Can you work these out from the model? Positions are in its coordinate system, mm. A direction names the side the tool comes from. Give positions to 0.01 mm unless a question says otherwise; leave off trailing zeros. Answer as a JSON object with one key per item and string values.
```python
from build123d import *

# Parameters (mm, degrees)
SKETCH1_W                = 127
SKETCH1_H                = 57.15
BOSS_EXTRUDE1_DEPTH      = 6.35
BOSS_EXTRUDE2_DEPTH      = 22.225
BOSS_EXTRUDE2_DEPTH_BACK = 22.225
SKETCH3_R                = 22.225
SKETCH4_R                = 12.7
CUT_EXTRUDE2_DEPTH       = 83.611035128
CUT_EXTRUDE2_DRAFT       = -7.5
BOSS_EXTRUDE3_DEPTH      = 6.35
CHAMFER1_SIZE            = 3.175
CHAMFER1_SIZE2           = 3.687920954
FILLET1_R                = 2.0955


with BuildPart() as part:
    # Sketch1 → Boss-Extrude1 (new body)
    with BuildSketch(Plane(origin=(0, 0, 0), x_dir=(1, 0, 0), z_dir=(0, 1, 0))):
        Rectangle(SKETCH1_W, SKETCH1_H)
    extrude(amount=BOSS_EXTRUDE1_DEPTH)

    # Cut-Extrude1 cone 1 section (through the dimple's axis) → Cut-Extrude1 (revolve, cut)
    with BuildSketch(Plane(origin=(-50.8, 6.35, 0), x_dir=(0, 0, 1), z_dir=(1, 0, 0))):
        Polygon((0, 0), (4.7625, 0), (0, 17.773891971), align=None)
    revolve(axis=Axis((-50.8, 6.35, 0), (0, -1, 0)), mode=Mode.SUBTRACT)

    # Cut-Extrude1 cone 2 section (through the dimple's axis) → Cut-Extrude1 cone 2 (revolve, cut)
    with BuildSketch(Plane(origin=(50.8, 6.35, 0), x_dir=(0, 0, 1), z_dir=(1, 0, 0))):
        Polygon((0, 0), (4.7625, 0), (0, 17.773891971), align=None)
    revolve(axis=Axis((50.8, 6.35, 0), (0, -1, 0)), mode=Mode.SUBTRACT)

    # Sketch3 → Boss-Extrude2 (add, two sides: drawn at the far end of the back side and taken through both)
    with BuildSketch(Plane(origin=(0, 6.35, 0), x_dir=(1, 0, 0), z_dir=(0, 1, 0)).offset(-BOSS_EXTRUDE2_DEPTH_BACK)):
        with Locations(Location((0, 0, 0), (0, 0, 270))):
            Circle(SKETCH3_R)
    extrude(amount=BOSS_EXTRUDE2_DEPTH + BOSS_EXTRUDE2_DEPTH_BACK)


with BuildPart() as cut_extrude2_tool:
    # Sketch4 → Cut-Extrude2 (with draft: the straight prism first)
    with BuildSketch(Plane(origin=(0, 28.575, 0), x_dir=(1, 0, 0), z_dir=(0, 1, 0))):
        Circle(SKETCH4_R)
    extrude(amount=-CUT_EXTRUDE2_DEPTH)
    # Cut-Extrude2: the draft: its side faces are tilted about the plane it starts from
    cut_extrude2_sides = [cut_extrude2_tool.faces().sort_by_distance(p)[0] for p in [
        (-12.7, -13.230517564, 0),
    ]]
    draft(cut_extrude2_sides, Plane(origin=(0, 28.575, 0), x_dir=(1, 0, 0), z_dir=(0, 1, 0)), CUT_EXTRUDE2_DRAFT)


with BuildPart() as part_1:
    add(part.part)

    # Cut-Extrude2: cut by cut_extrude2_tool
    add(cut_extrude2_tool.part, mode=Mode.SUBTRACT)

    # Sketch5 → Boss-Extrude3 (add)
    with BuildSketch(Plane.XY.offset(19.05)):
        Polygon((11.43, 22.225), (11.43, 6.35), (60.325, 6.35), align=None)
        Polygon((-11.43, 22.225), (-11.43, 6.35), (-60.325, 6.35), align=None)
    boss_extrude3 = extrude(amount=-BOSS_EXTRUDE3_DEPTH)

    # Mirror1: Boss-Extrude3 across plane
    add(boss_extrude3.mirror(Plane.XY))

    # Chamfer1
    chamfer1_edges = [part_1.edges().sort_by_distance(p)[0] for p in [
        (-12.7, 28.575, 0),
    ]]
    chamfer1_side = [part_1.faces().sort_by_distance(p)[0] for p in [
        (0, 28.575, -21.596382072),
    ]]
    chamfer(chamfer1_edges, length=CHAMFER1_SIZE, length2=CHAMFER1_SIZE2, reference=chamfer1_side[0])

    # Fillet1
    fillet1_edges = [part_1.edges().sort_by_distance(p)[0] for p in [
        (35.88631265, 14.28463875, 19.05),
        (39.281993201, 13.182145064, 12.7),
        (35.88631265, 14.28463875, -19.05),
        (39.281993201, 13.182145064, -12.7),
        (-39.281993201, 13.182145064, 12.7),
        (-35.88631265, 14.28463875, 19.05),
        (-39.281993201, 13.182145064, -12.7),
        (-35.88631265, 14.28463875, -19.05),
        (-22.225, 6.35, 0),
        (5.939881102, 6.35, 21.416545882),
        (22.225, 6.35, 0),
        (0, 6.35, -22.225),
        (-63.5, 6.35, 0),
        (-63.5, 0, 0),
        (0, 6.35, -28.575),
        (-63.5, 3.175, -28.575),
        (0, 0, -28.575),
        (63.5, 6.35, 0),
        (63.5, 3.175, -28.575),
        (63.5, 0, 0),
        (-63.5, 3.175, 28.575),
        (0, 6.35, 28.575),
        (63.5, 3.175, 28.575),
        (0, 0, 28.575),
        (0, 28.575, -22.225),
    ]]
    fillet(fillet1_edges, radius=FILLET1_R)


solid = part_1.part
```
1) If we mould it in two halves opening along Z, with no side actions, what happens to faces 4 (the flat face through (37.669, 13.706, 15.89)), 5 (the cylindrical face through (35.65, 13.7, 18.45)), 6 (the flat face through (28, 10, 12.7))? For each: +Z half, -Z half, draft (parallel to the pull), parting line (faces both ways), or undercut.
Answer list:
{"face 4": "draft", "face 5": "+Z half", "face 6": "undercut"}
2) Please list where these lines run through material, in increasing order: line 1 along Z through (x, y) = (-20.5, 13); line 2 along Y through (x, z) = (-52, 6); line 3 along X through (y, z) = (-1, -2.5). Write a range as from..to.
Answer list:
{"line 1": "-19.05..-12.7, -8.58..8.58, 12.7..19.05", "line 2": "0..6.35", "line 3": "-22.08..-8.44, 8.44..22.08"}
3) For faces 1 (the flat face through (-23, 10, -19.05)), 2 (the cylindrical face through (18.74, -8.05, 11.95)), 3 (the cylindrical face through (37.954, 12.951, -13.298)), which set-ups out of +Z, -Z, +X, -X, +Y, -Y let a thin tool reach every point of the face, with its end or its side?
Answer list:
{"face 1": "-Z, -X, +Y", "face 2": "-Y", "face 3": "+X, +Y"}
4) Will these pins go through, and if not, where does the flat tip stop? pin 1 Ø5.5 at (x, y) = (36.5, 11.5) entering from +Z; pin 2 Ø12.5 at (x, y) = (-42, 11) entering from +Z; pin 3 Ø15 at (x, y) = (32.5, 13) entering from -Z; pin 4 Ø15 at (x, y) = (-25, 11.5) entering from +Z (3 decimals).
Answer list:
{"pin 1": "z = 19.05", "pin 2": "z = 28.52", "pin 3": "z = -28.16", "pin 4": "z = 28.575"}
5) Suppose I cut it at A-A, the plane z = 0. Give the number of separate pieces and of enclosed holes in the cut face, and give its area (3 significant figures).
Answer list:
{"separate pieces": "4", "enclosed holes": "0", "area": "1,520 mm^2"}
